For this review, use the dimensioned drawing (mm, ordinates from the lowest corner) and the shaded views. Give positions to 0.01 mm unless a question says otherwise; leave off trailing zeros. Loops run counter-clockwise (first coordinate to the right, second up) from the corner with the lowest first, then second, coordinate; pieces in that order, holes last. Notation, with made-up numbers: (16.5, 33) -> (61.5, 33) arc R26 cw to (61.5, 70) -> close; hole circle Ø9 at (-19.5, 43). An arc over 180 degrees is marked (long way). Use a Markdown table: item, result. Add a question column.
1. For pin 1 Ø4.5 at (x, y) = (10.16, 3.81) entering from -Z; pin 2 Ø5.5 at (x, y) = (47.47, 27.58) entering from -Z, all flat-tipped, find the tip position at first contact; note any pin that passes through.
2. Draft analysis for pull direction X (two halves, no side actions). For the marked faces 1, 2 and 3, state which applies: pulls with the +X half, pulls with the -X half, needs draft (parallel to the pull), parting line crosses it, or undercut.
3. Add section D-D (x = 55.88). State the section outline as (y, z) points.
4. Add section B-B (x = 10.16). State the section outline as (y, z) points, and give its area (3 significant figures).
5. To check wall thickness, follow line 1 (Y direction, x = 63.5, z = 4.25); line 2 (X direction, y = 24, z = 3.75) (1 decimal); line 3 (Y direction, x = 65, z = 5.75) (1 decimal). State the ranges of each line that lie inside material, in increasing order.
6. Add section C-C (y = 59.69). State the section outline as (x, z) points.
7. Add section A-A (y = 3.81). State the section outline as (x, z) points.
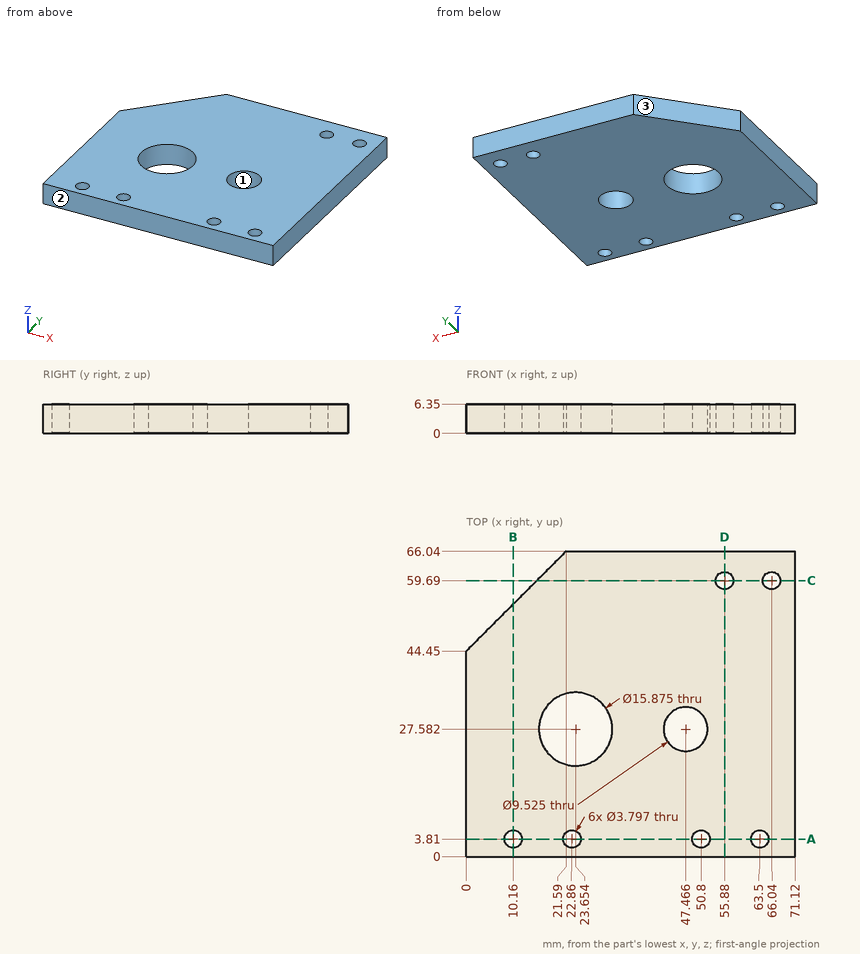
Taken from the geometry:
| question | item | result |
|---|---|---|
| 1 | pin 1 | stops at z = 0 |
| 1 | pin 2 | passes through |
| 2 | face 1 | undercut |
| 2 | face 2 | needs draft |
| 2 | face 3 | pulls with the -X half |
| 3 | outline | (0, 0) -> (57.79, 0) -> (57.79, 6.35) -> (0, 6.35) -> close; (61.59, 0) -> (66.04, 0) -> (66.04, 6.35) -> (61.59, 6.35) -> close |
| 4 | outline | (0, 0) -> (1.91, 0) -> (1.91, 6.35) -> (0, 6.35) -> close; (5.71, 0) -> (54.61, 0) -> (54.61, 6.35) -> (5.71, 6.35) -> close |
| 4 | area | 323 mm^2 |
| 5 | line 1 | y = 0 to 1.91, 5.71 to 66.04 |
| 5 | line 2 | x = 0 to 16.6, 30.7 to 44.3, 50.6 to 71.1 |
| 5 | line 3 | y = 0 to 2.6, 5 to 58.1, 61.3 to 66 |
| 6 | outline | (15.24, 0) -> (53.98, 0) -> (53.98, 6.35) -> (15.24, 6.35) -> close; (57.78, 0) -> (64.14, 0) -> (64.14, 6.35) -> (57.78, 6.35) -> close; (67.94, 0) -> (71.12, 0) -> (71.12, 6.35) -> (67.94, 6.35) -> close |
| 7 | outline | (0, 0) -> (8.26, 0) -> (8.26, 6.35) -> (0, 6.35) -> close; (12.06, 0) -> (20.96, 0) -> (20.96, 6.35) -> (12.06, 6.35) -> close; (24.76, 0) -> (48.9, 0) -> (48.9, 6.35) -> (24.76, 6.35) -> close; (52.7, 0) -> (61.6, 0) -> (61.6, 6.35) -> (52.7, 6.35) -> close; (65.4, 0) -> (71.12, 0) -> (71.12, 6.35) -> (65.4, 6.35) -> close |
